Autodesk Inventor part; units mm, degrees
ref_plane "YZ Plane" through (0, 0, 0) normal (1, 0, 0) x (0, 1, 0)
ref_plane "XZ Plane" through (0, 0, 0) normal (0, 1, 0) x (-1, 0, 0)
ref_plane "XY Plane" through (0, 0, 0) normal (0, 0, 1) x (1, 0, 0)
sketch "Sketch1" plane through (0, 0, 0) normal (0, 0, 1) x (1, 0, 0)
  circle A0 centre (0, 0) radius 55
  circle A1 centre (0, 0) radius 10
  dimension "d0" = 110
  dimension "d1" = 20
extrude "Extrusion1" add sketch "Sketch1" along normal blind 4
sketch "Sketch2" plane through (0, 0, 4) normal (0, 0, 1) x (1, 0, 0)
  point P0 (0, 0)
  point P1 (0, 34)
  point P2 (-29.4449, 17)
  point P3 (-29.4449, -17)
  point P4 (0, -34)
  point P5 (29.4449, -17)
  point P6 (29.4449, 17)
  dimension "d4" = 34
  dimension "d7" = 360
hole "Hole1" at (0, 34, 4) at (-29.4449, 17, 4) at (-29.4449, -17, 4) at (0, -34, 4) at (29.4449, -17, 4) at (29.4449, 17, 4) direction (0, 0, -1) diameter 32.5 end through all
sketch "Sketch3" plane through (0, 0, 4) normal (0, 0, 1) x (1, 0, 0)
  point P0 (0, 0)
  point P1 (22, 40)
  point P2 (-23.641, 39.0526)
  point P3 (-45.641, -0.9474)
  point P4 (-22, -40)
  point P5 (23.641, -39.0526)
  point P6 (45.641, 0.9474)
  dimension "d18" = 360
hole "Hole2" at (22, 40, 4) at (-23.641, 39.0526, 4) at (-45.641, -0.9474, 4) at (-22, -40, 4) at (23.641, -39.0526, 4) at (45.641, 0.9474, 4) direction (0, 0, -1) diameter 5 end through all
equation "\"d14\" = Thickness"
equation "\"BendRadius\" = Thickness"
equation "\"BendReliefWidth\" = Thickness"
equation "\"BendReliefDepth\" = 0.5 * Thickness"
equation "\"CornerReliefSize\" = 4 * Thickness"
equation "\"MinimumRemnant\" = 2 * Thickness"
equation "\"TransitionRadius\" = BendRadius"
equation "\"JacobiRadiusSize\" = BendRadius"
equation "\"GapSize\" = Thickness"
properties part number "Electromagnetic cover bottom"
Design review of the part built by this model. Coordinates are the model's own, in mm. Round coordinates to 2 decimals unless told otherwise and drop trailing zeros. Loops run counter-clockwise (first coordinate to the right, second up) from the corner with the lowest first, then second, coordinate; pieces in that order, holes last. Notation, with made-up numbers: (4.25, 46.5) - (60.25, 46.5) arc R5 cw to (60.25, 52.5) - close; hole circle Ø7 at (-31.75, 45). An arc over 180 degrees is marked (long way). One line per question, with ' | ' between items.
1. We need section C-C, the plane y = 6. State the section outline as (x, z) points.
Results are:
outline: (-54.67, 0) - (-41.41, 0) - (-41.41, 4) - (-54.67, 4) - close; (-17.48, 0) - (-8, 0) - (-8, 4) - (-17.48, 4) - close; (8, 0) - (17.48, 0) - (17.48, 4) - (8, 4) - close; (41.41, 0) - (54.67, 0) - (54.67, 4) - (41.41, 4) - close
2. For L1, parallel to X at y = 17, z = 2.75; L2, parallel to Y at x = 9, z = 2.6; L3, parallel to Y at x = -18, z = 3.3, list the stretches that pass through material, from the lowest coordinate up. Write a range as [from, to].
Results are:
L1: x = [-52.31, -45.69], [-13.19, 13.19], [45.69, 52.31] | L2: y = [-54.26, -47.53], [-20.47, -4.36], [4.36, 20.47], [47.53, 54.26] | L3: y = [-51.97, -28.54], [-5.46, 5.46], [28.54, 51.97]
3. We need section A-A, the plane x = 0. State the section outline as (y, z) points.
Results are:
outline: (-55, 0) - (-50.25, 0) - (-50.25, 4) - (-55, 4) - close; (-17.75, 0) - (-10, 0) - (-10, 4) - (-17.75, 4) - close; (10, 0) - (17.75, 0) - (17.75, 4) - (10, 4) - close; (50.25, 0) - (55, 0) - (55, 4) - (50.25, 4) - close
4. We need section D-D, the plane x = -18. State the section outline as (y, z) points, and give its area (3 significant figures).
Results are:
outline: (-51.97, 0) - (-28.54, 0) - (-28.54, 4) - (-51.97, 4) - close; (-5.46, 0) - (5.46, 0) - (5.46, 4) - (-5.46, 4) - close; (28.54, 0) - (51.97, 0) - (51.97, 4) - (28.54, 4) - close | area: 231 mm²
5. We need section B-B, the plane y = -48. State the section outline as (x, z) points.
Results are:
outline: (-26.85, 0) - (-8.25, 0) - (-8.25, 4) - (-26.85, 4) - close; (8.25, 0) - (26.85, 0) - (26.85, 4) - (8.25, 4) - close
6. Draft analysis for pull direction Y (two halves, no side actions). For faces 1 (the face through (-1, -11, 4)), 2 (the face through (-11.923, 53.692, 1.972)), 3 (the face through (-24.11, -41.34, 1.97)), state which applies: released by +Y, released by -Y, zero draft, split by the parting line, or undercut.
Results are:
face 1: zero draft | face 2: split by the parting line | face 3: undercut
